Build history of the part. All positions in model axes, mm. A direction names the side the tool comes from. Give positions to 0.01 mm unless a question says otherwise; leave off trailing zeros. Write each loop counter-clockwise with the first axis right and the second up, starting at its lowest first coordinate (ties: lowest second). Pieces come first, ordered by that corner, then holes.
Autodesk Inventor part; units mm, degrees
ref_plane "YZ Plane" through (0, 0, 0) normal (1, 0, 0) x (0, 1, 0)
ref_plane "XZ Plane" through (0, 0, 0) normal (0, 1, 0) x (-1, 0, 0)
ref_plane "XY Plane" through (0, 0, 0) normal (0, 0, 1) x (1, 0, 0)
sketch "Sketch1" plane through (0, 0, 0) normal (1, 0, 0) x (0, 1, 0)
  line L0 (482.3395, 530.3412) -> (-338.3345, 530.3412)
  line L1 (-338.3345, 530.3412) -> (-338.3345, -174.5088)
  line L2 (-338.3345, -174.5088) -> (482.3395, -174.5088)
  line L3 (482.3395, -174.5088) -> (482.3395, 530.3412)
  point P0 (0, 0)
  dimension "d0" = 820.674
  dimension "d1" = 704.85
extrude "Extrusion1" add sketch "Sketch1" along normal blind 127
sketch "Sketch2" plane through (127, 0, 0) normal (1, 0, 0) x (0, 0, -1)
  line L0 (174.5088, 482.3395) -> (-530.3412, 482.3395)
  line L1 (-530.3412, -338.3345) -> (174.5088, -338.3345)
  line L2 (-530.3412, 482.3395) -> (-454.1412, 482.3395)
  line L3 (-454.1412, 482.3395) -> (-454.1412, -338.3345)
  line L4 (-454.1412, -338.3345) -> (-530.3412, -338.3345)
  line L5 (-530.3412, -338.3345) -> (-530.3412, 482.3395)
  line L6 (174.5088, 482.3395) -> (98.3088, 482.3395)
  line L7 (98.3088, 482.3395) -> (98.3088, -338.3345)
  line L8 (98.3088, -338.3345) -> (174.5088, -338.3345)
  line L9 (174.5088, -338.3345) -> (174.5088, 482.3395)
  line L10 (174.5088, -338.3345) -> (174.5088, 482.3395)
  point P0 (0, 0)
  dimension "d4" = 76.2
  dimension "d5" = 76.2
  dimension "d6" = 0
extrude "Extrusion2" add sketch "Sketch2" along normal blind 25.4 contours L9 L1 L7 L0 | L3 L1 L5 L0
sketch "Sketch3" plane through (127, 0, 0) normal (1, 0, 0) x (0, 0, -1)
  line L0 (-454.1412, 482.3395) -> (-454.1412, -338.3345)
  line L1 (-352.5412, 101.3395) -> (-454.1412, 101.3395)
  line L2 (-454.1412, 101.3395) -> (-454.1412, -0.2605)
  line L3 (-454.1412, -0.2605) -> (-352.5412, -0.2605)
  line L4 (-352.5412, -0.2605) -> (-352.5412, 101.3395)
  line L5 (98.3088, -338.3345) -> (98.3088, 482.3395)
  line L6 (-3.2912, 101.3395) -> (98.3088, 101.3395)
  line L7 (98.3088, 101.3395) -> (98.3088, -0.2605)
  line L8 (98.3088, -0.2605) -> (-3.2912, -0.2605)
  line L9 (-3.2912, -0.2605) -> (-3.2912, 101.3395)
  line L10 (98.3088, 482.3395) -> (-454.1412, 482.3395)
  point P0 (0, 0)
  dimension "d9" = 101.6
  dimension "d10" = 101.6
  dimension "d11" = 101.6
  dimension "d12" = 101.6
  dimension "d13" = 381
extrude "Extrusion3" add sketch "Sketch3" along normal blind 25.4
properties part number "BlockBase"
1. Drop flat-ended pins along their axis: pin 1 (12 mm diameter, centred on y = 199, z = 2.5, fed in from +X); pin 2 (20.5 mm diameter, centred on x = 135.5, z = 385.5, fed in from -Y); pin 3 (20.5 mm diameter, centred on x = 138.5, z = 404, fed in from +Y). Give the stop position or say it passes through.
2. Drill centre lines: line 1 along Z through (x, y) = (138, -206); line 2 along X through (y, z) = (-105, 215.5). Where is each one in solid material? Low to high.
3. Saw through at A-A on x = 141.5. Give the cut face in (y, z), plus the area to 3 significant figures.
4. Saw through at D-D on z = 326.5. Give the cut face in (x, y), plus the area to 3 significant figures.
5. 3-axis set-ups, long thin cutter, end or side, ignore diameter. For faces 4 (the face through (140, -167, 454.141)), 5 (the face through (0, 66, 183)), 6 (the face through (140, 295, -98.309)), 7 (the face through (75, 78, 530.341)), 8 (the face through (140, 50, 352.541)): which of +Z, -Z, +X, -X, +Y, -Y reach the whole face in a straight line?
6. Saw through at B-B on y = 16. Give the cut face in (x, z), plus the area to 3 significant figures.
7. Saw through at C-C on z = 445. Give the cut face in (x, y).
8. Mould opens along Z. For faces 1 (the face through (140, -167, -98.309)), 2 (the face through (75, -338.334, 183)), 3 (the face through (75, 66, -174.509)) say: pulls with the +Z half, pulls with the -Z half, needs draft (parallel to the pull), parting line crosses it, or undercut.
Outcome:
1. pin 1: stops at x = 127
1. pin 2: stops at y = -338.33
1. pin 3: stops at y = 101.34
2. line 1: z = -174.51 to -98.31, 454.14 to 530.34
2. line 2: x = 0 to 127
3. outline: (-338.33, -174.51) - (482.34, -174.51) - (482.34, -98.31) - (101.34, -98.31) - (101.34, 3.29) - (-0.26, 3.29) - (-0.26, -98.31) - (-338.33, -98.31) - close; (-338.33, 454.14) - (-0.26, 454.14) - (-0.26, 352.54) - (101.34, 352.54) - (101.34, 454.14) - (482.34, 454.14) - (482.34, 530.34) - (-338.33, 530.34) - close
3. area: 146,000 mm2
4. outline: (0, -338.33) - (127, -338.33) - (127, 482.34) - (0, 482.34) - close
4. area: 104,000 mm2
5. face 4: +X, -Y
5. face 5: +Z, -Z, -X, +Y, -Y
5. face 6: +X, +Y
5. face 7: +Z, +X, -X, +Y, -Y
5. face 8: +X, +Y, -Y
6. outline: (0, -174.51) - (152.4, -174.51) - (152.4, 3.29) - (127, 3.29) - (127, 352.54) - (152.4, 352.54) - (152.4, 530.34) - (0, 530.34) - close
6. area: 98,500 mm2
7. outline: (0, -338.33) - (127, -338.33) - (127, -0.26) - (152.4, -0.26) - (152.4, 101.34) - (127, 101.34) - (127, 482.34) - (0, 482.34) - close
8. face 1: undercut
8. face 2: needs draft
8. face 3: pulls with the -Z half
